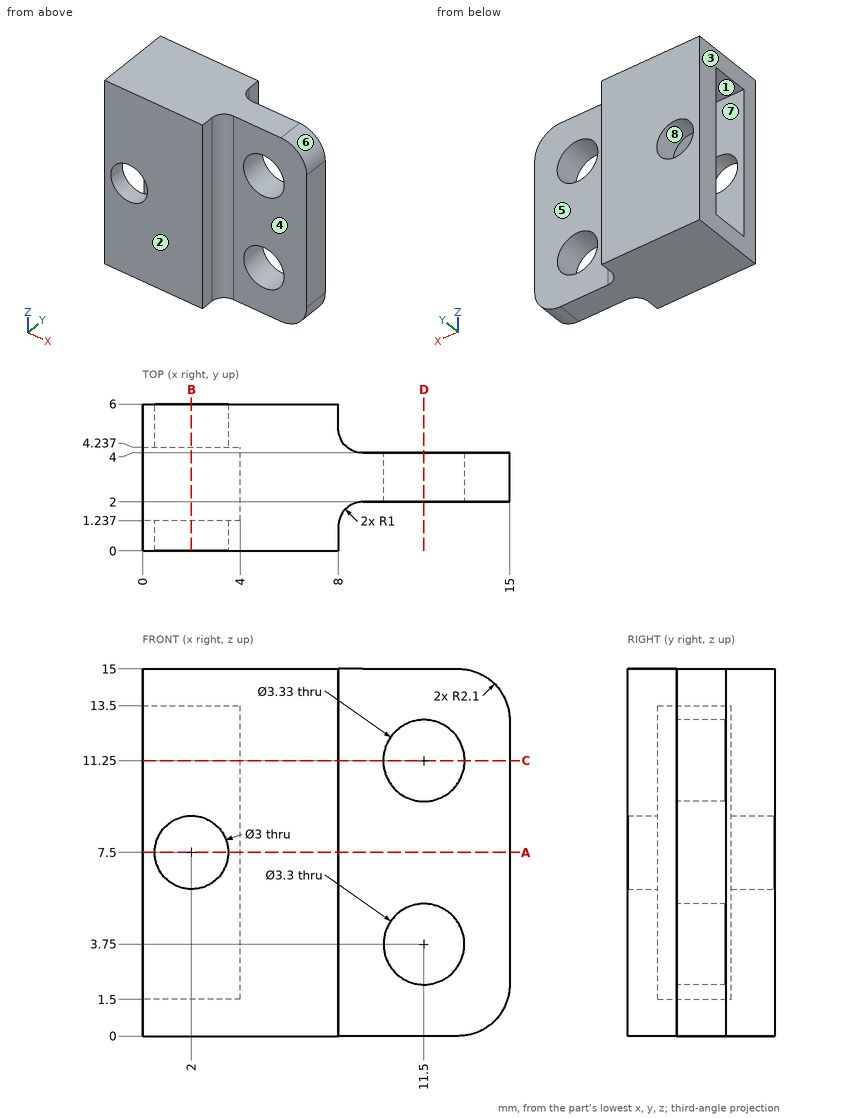
Drawing for the job (mm, zero at the part's lowest x, y, z). A direction names the side the tool comes from. Give positions to 0.01 mm unless a question says otherwise; leave off trailing zeros. Loops run counter-clockwise (first coordinate to the right, second up) from the corner with the lowest first, then second, coordinate; pieces in that order, holes last.
Item 1: Slice it at D-D (x = 11.5). Write the cut outline in (y, z) (3 decimals).
Check values:
outline: (2, 0) - (4, 0) - (4, 2.1) - (2, 2.1) - close; (2, 5.4) - (4, 5.4) - (4, 9.585) - (2, 9.585) - close; (2, 12.915) - (4, 12.915) - (4, 15) - (2, 15) - close
Item 2: Which spindle directions (+Z, -Z, +X, -X, +Y, -Y) get a long thin tool onto all of the face, cutting with end or side? Do the marked faces 1, 2, 3, 4 and 5. Say none if no direction does.
Check values:
face 1: -X
face 2: +Z, -Z, +X, -X, -Y
face 3: +Z, -Z, -X, +Y, -Y
face 4: +Z, -Z, +X, -Y
face 5: +Z, -Z, +X, +Y
Item 3: Slice it at A-A (z = 7.5). Write the cut outline in (x, y), plus the area to 3 significant figures.
Check values:
outline: (0, 0) - (0.5, 0) - (0.5, 1.24) - (0, 1.24) - close; (0, 4.24) - (0.5, 4.24) - (0.5, 6) - (0, 6) - close; (3.5, 0) - (8, 0) - (8, 1) arc R1 cw to (9, 2) - (15, 2) - (15, 4) - (9, 4) arc R1 cw to (8, 5) - (8, 6) - (3.5, 6) - (3.5, 4.24) - (4, 4.24) - (4, 1.24) - (3.5, 1.24) - close
area: 41.4 mm2
Item 4: Slice it at C-C (z = 11.25). Write the cut outline in (x, y) (1 decimal), plus the area to 3 significant figures.
Check values:
outline: (0, 0) - (8, 0) - (8, 1) arc R1 cw to (9, 2) - (9.8, 2) - (9.8, 4) - (9, 4) arc R1 cw to (8, 5) - (8, 6) - (0, 6) - (0, 4.2) - (4, 4.2) - (4, 1.2) - (0, 1.2) - close; (13.2, 2) - (15, 2) - (15, 4) - (13.2, 4) - close
area: 43.8 mm2
Item 5: Slice it at B-B (x = 2). Write the cut outline in (y, z).
Check values:
outline: (0, 0) - (6, 0) - (6, 6) - (4.24, 6) - (4.24, 1.5) - (1.24, 1.5) - (1.24, 6) - (0, 6) - close; (0, 9) - (1.24, 9) - (1.24, 13.5) - (4.24, 13.5) - (4.24, 9) - (6, 9) - (6, 15) - (0, 15) - close
Item 6: Drill centre lines: line 1 along Z through (x, y) = (11.5, 3.4) (3 decimals); line 2 along Z through (x, y) = (10.75, 2.6); line 3 along Z through (x, y) = (3, 3.9). Where is each one in solid material? Low to high.
Check values:
line 1: z = 0 to 2.1, 5.4 to 9.585, 12.915 to 15
line 2: z = 0 to 2.28, 5.22 to 9.76, 12.74 to 15
line 3: z = 0 to 1.5, 13.5 to 15
Item 7: Mould opens along X. For the marked faces 6, 7 and 8 say: +X half, -X half, draft (parallel to the pull), parting line (faces both ways), or undercut.
Check values:
face 6: +X half
face 7: draft
face 8: undercut
Item 8: Drop flat-ended pins along their axis: P1, Ø1.8, axis at x = 12, z = 5.5, coming from the -Y side; P2, Ø0.5, axis at y = 0.5, z = 7.5, coming from the +X side; P3, Ø5, axis at x = 11, z = 11, coming from the -Y side. Give the stop position or say it passes through.
Check values:
P1: stops at y = 2
P2: stops at x = 8
P3: stops at y = 1.87
